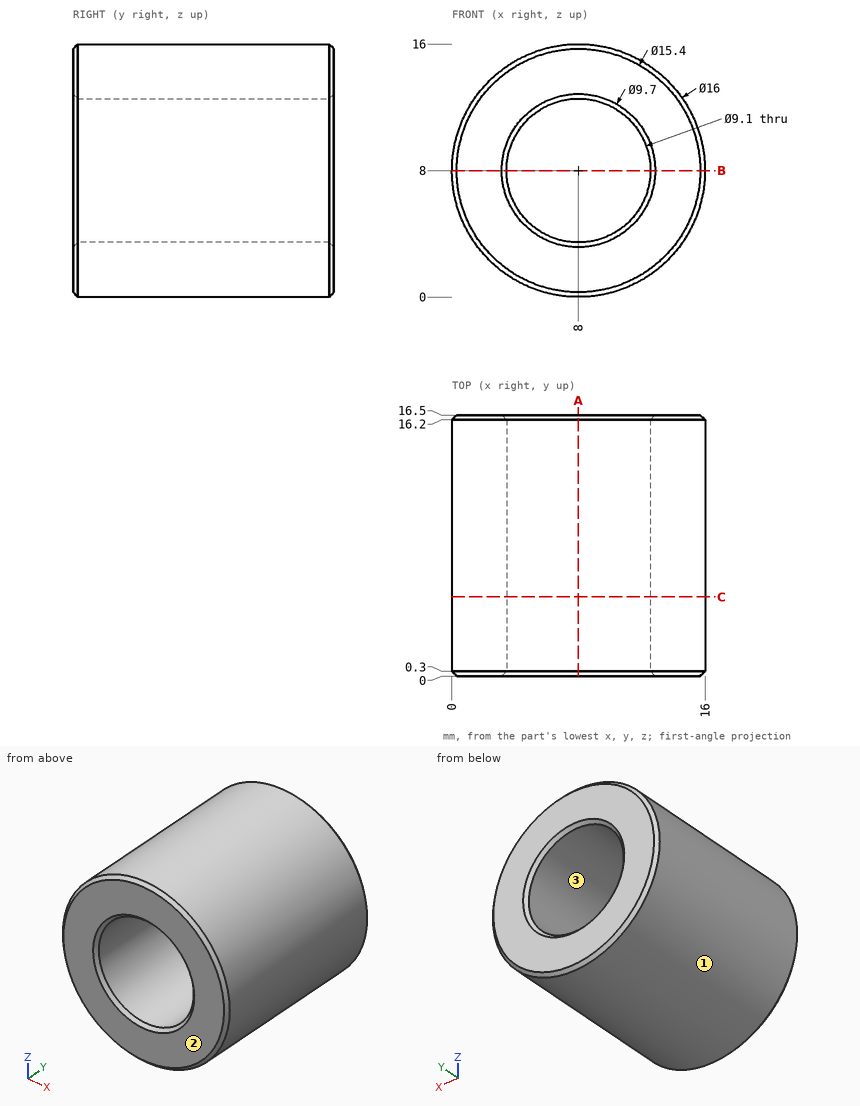
The drawing under review shows one solid part. Ordinate dimensions are in mm from its lowest x, y, z. Coordinates: 2 decimals unless noted, no trailing zeros. Order: outer loops, then holes, each group sorted by start corner. A loop starts at its lowest first (then second) coordinate and runs counter-clockwise, first axis right, second up. Notation, with made-up numbers: M 7.25,56 L 21.25,56 A27 ccw 21.25,91 Z; hole C 10,63 d9. An arc over 180 degrees is marked long. Use a Markdown table: item, result.
(1) For P1, Ø3, axis at y = 11.5, z = 4.5, coming from the -X side; P2, Ø2, axis at y = 14.5, z = 2.5, coming from the +X side; P3, Ø2, axis at y = 12, z = 9.5, coming from the -X side, all flat-tipped, find the tip position at first contact; note any pin that passes through.
Worked answers:
| item | result |
|---|---|
| P1 | stops at x = 0.25 |
| P2 | stops at x = 14.61 |
| P3 | stops at x = 0.02 |
(2) Draft analysis for pull direction Z (two halves, no side actions). For the marked faces 1, 2 and 3, state which applies: released by +Z, released by -Z, zero draft, split by the parting line, or undercut.
Worked answers:
| item | result |
|---|---|
| face 1 | split by the parting line |
| face 2 | zero draft |
| face 3 | undercut |
(3) Add section C-C (y = 5). Give the boundary of the cut face in (x, z).
Worked answers:
| item | result |
|---|---|
| outline | C 8,8 d16; hole C 8,8 d9.1 |
(4) Add section A-A (x = 8). Give the boundary of the cut face in (y, z).
Worked answers:
| item | result |
|---|---|
| outline | M 0,0.3 L 0.3,0 L 16.2,0 L 16.5,0.3 L 16.5,3.15 L 16.2,3.45 L 0.3,3.45 L 0,3.15 Z; M 0,12.85 L 0.3,12.55 L 16.2,12.55 L 16.5,12.85 L 16.5,15.7 L 16.2,16 L 0.3,16 L 0,15.7 Z |
(5) Add section B-B (z = 8). Give the boundary of the cut face in (x, y), then the cut area to 3 significant figures.
Worked answers:
| item | result |
|---|---|
| outline | M 0,0.3 L 0.3,0 L 3.15,0 L 3.45,0.3 L 3.45,16.2 L 3.15,16.5 L 0.3,16.5 L 0,16.2 Z; M 12.55,0.3 L 12.85,0 L 15.7,0 L 16,0.3 L 16,16.2 L 15.7,16.5 L 12.85,16.5 L 12.55,16.2 Z |
| area | 113 mm2 |
(6) Wall thickness on probe 1 along X at (y, z) = (12.75, 8); probe 2 along X at (y, z) = (3, 4.75); probe 3 along Z at (x, y) = (6, 11.5): over which ranges is each line inside the solid? List them lowest first.
Worked answers:
| item | result |
|---|---|
| probe 1 | x = 0 to 3.45, 12.55 to 16 |
| probe 2 | x = 0.69 to 4.82, 11.18 to 15.31 |
| probe 3 | z = 0.25 to 3.91, 12.09 to 15.75 |
